Autodesk Inventor part; units mm, degrees
ref_plane "YZ Plane" through (0, 0, 0) normal (1, 0, 0) x (0, 1, 0)
ref_plane "XZ Plane" through (0, 0, 0) normal (0, 1, 0) x (-1, 0, 0)
ref_plane "XY Plane" through (0, 0, 0) normal (0, 0, 1) x (1, 0, 0)
sketch "Sketch1" plane through (0, 0, 0) normal (0, 0, 1) x (1, 0, 0)
  line L0 (-59.5, -59.5) -> (59.5, -59.5)
  line L1 (59.5, -59.5) -> (59.5, 59.5)
  line L2 (59.5, 59.5) -> (-59.5, 59.5)
  line L3 (-59.5, 59.5) -> (-59.5, -59.5)
  line L4 (-59.5, -59.5) -> (59.5, 59.5) construction
  line L5 (59.5, -59.5) -> (-59.5, 59.5) construction
  circle A0 centre (-52.4, 52.4) radius 2.25
  circle A1 centre (52.4, 52.4) radius 2.25
  line L6 (-23.2863, -58) -> (23.2863, -58)
  line L7 (58, -23.2863) -> (58, 23.2863)
  line L8 (23.2863, 58) -> (-23.2863, 58)
  line L9 (-58, 23.2863) -> (-58, -23.2863)
  line L10 (-58, -58) -> (58, 58) construction
  line L11 (58, -58) -> (-58, 58) construction
  arc A2 (-58, -23.2863) -> (-23.2863, -58) centre (0, 0) ccw
  arc A3 (23.2863, -58) -> (58, -23.2863) centre (0, 0) ccw
  arc A4 (58, 23.2863) -> (23.2863, 58) centre (0, 0) ccw
  arc A5 (-23.2863, 58) -> (-58, 23.2863) centre (0, 0) ccw
  arc A6 (-52.4, 59.5) -> (-59.5, 52.4) centre (-52.4, 52.4) ccw
  dimension "d0" = 119
  dimension "d2" = 4.5
  dimension "d3" = 104.8
  dimension "d5" = 116
  dimension "d6" = 62.5
  dimension "d7" = 46.5725
  dimension "d15" = 1.5
extrude "Extrusion1" add sketch "Sketch1" along normal blind 38 contours L3 A6 L2 L1 L0 | L3 L2 A6 | A0 | A1
extrude "Extrusion2" cut sketch "Sketch1" along normal blind 38 contours L3 L2 A6 | A0
pattern_circular "Circular Pattern1" count 4 over 360 about axis through (0, 0, 0) along (0, 0, 1) of "Extrusion2"
equation "\"d0\" = length"
equation "\"d2\" = holeSize"
equation "\"d3\" = dHoles"
equation "\"d5\" = fanCutOff"
equation "\"d6\" = 0.5 * fanDia"
equation "\"d8\" = heigth"
equation "\"d10\" = heigth"
equation "\"length\" = 119"
equation "\"width\" = length"
equation "\"heigth\" = 38"
equation "\"dHoles\" = 104.8"
equation "\"holeSize\" = 4.5"
equation "\"fanDia\" = 125"
equation "\"fanCutOff\" = 116"
equation "\"d4\" = fanDia"
properties part number "120mm Fan"
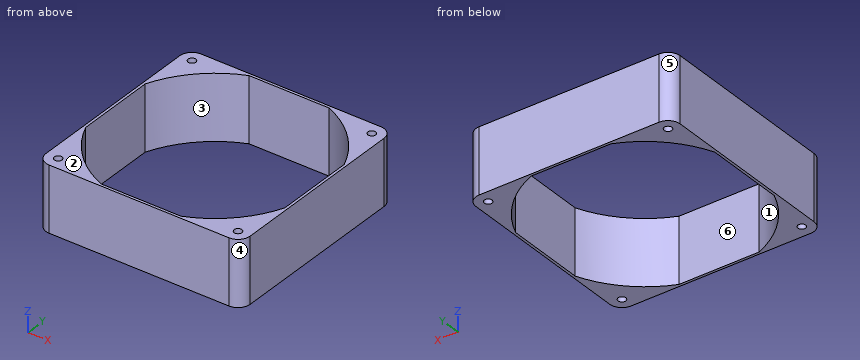
Geometry check sheet. Reference: the model listing, model coordinates, mm. Face numbers are marked on the shaded views. A direction names the side the tool comes from. Give positions to 0.01 mm unless a question says otherwise; leave off trailing zeros. Loops run counter-clockwise (first coordinate to the right, second up) from the corner with the lowest first, then second, coordinate; pieces in that order, holes last. Notation, with made-up numbers: M -17.5,50 L 40.5,50 A23 ccw 40.5,81 Z; hole C 39.5,25 d2. An arc over 180 degrees is marked long. Write item = value, one per line.
(1) Release check for a two-part mould opening along X. For the marked faces 3, 4, 5 and 6 record: released by +X, released by -X, zero draft, split by the parting line, or undercut.
Answer below:
face_3 = undercut
face_4 = released by +X
face_5 = released by -X
face_6 = undercut
(2) Gauge pin test, flat end, axial feed: pin 1 Ø5 at (x, y) = (-52.4, -52.4) entering from +Z. Record the tip position at first contact, or that the pin passes through.
Answer below:
pin_1 = 38
(3) Sectioned sample at B-B, the plane z = 26.5. Record the cut outline in (x, y).
Answer below:
outline = M -59.5,-52.4 A7.1 ccw -52.4,-59.5 L 52.4,-59.5 A7.1 ccw 59.5,-52.4 L 59.5,52.4 A7.1 ccw 52.4,59.5 L -52.4,59.5 A7.1 ccw -59.5,52.4 Z; hole M -58,-23.29 A62.5 ccw -23.29,-58 L 23.29,-58 A62.5 ccw 58,-23.29 L 58,23.29 A62.5 ccw 23.29,58 L -23.29,58 A62.5 ccw -58,23.29 Z; hole C -52.4,-52.4 d4.5; hole C -52.4,52.4 d4.5; hole C 52.4,-52.4 d4.5; hole C 52.4,52.4 d4.5
(4) Tool access check on the marked faces 1 and 2. Record the directions out of +Z, -Z, +X, -X, +Y, -Y that give a thin tool (end or side, any length) a straight path to the whole face; none if there is none.
Answer below:
face_1 = +Z, -Z
face_2 = +Z, +X, -X, +Y, -Y
(5) Sectioned sample at C-C, the plane x = -45. Record the cut outline in (y, z).
Answer below:
outline = M -59.5,0 L -43.37,0 L -43.37,38 L -59.5,38 Z; M 43.37,0 L 59.5,0 L 59.5,38 L 43.37,38 Z
(6) Sectioned sample at A-A, the plane y = -19. Record the cut outline in (x, z), plus the area to 3 significant figures.
Answer below:
outline = M -59.5,0 L -58,0 L -58,38 L -59.5,38 Z; M 58,0 L 59.5,0 L 59.5,38 L 58,38 Z
area = 114 mm2
(7) Material ranges on line 1 (Y direction, x = 8, z = 20); line 2 (X direction, y = -52, z = 20), recorded low to high. Write a range as [from, to].
Answer below:
line_1 = [-59.5, -58], [58, 59.5]
line_2 = [-59.5, -54.61], [-50.19, -34.67], [34.67, 50.19], [54.61, 59.5]
